Can you work these out from the drawing? Everything is in mm from the part's minimum corner. Give positions to 0.01 mm unless a question says otherwise; leave off trailing zeros. Write each question's results on one line, items separated by ' | '. Start each with the question number.
Item 1: Suppose I cut it at A-A on y = 1.25. Count the separate pieces of the cut face and the enclosed holes in it, then the cut area to 3 significant figures.
Item 2: Will these pins go through, and if not, where does the flat tip stop? P1, Ø2.5, axis at x = 15, z = 32.5, coming from the -Y side; P2, Ø5, axis at x = 109.015, z = 79, coming from the -Y side.
Item 3: Please list where these lines run through material, in increasing order: line 1 along Z through (x, y) = (100, 1.1); line 2 along X through (y, z) = (1.15, 32); line 3 along Z through (x, y) = (99, 0.85).
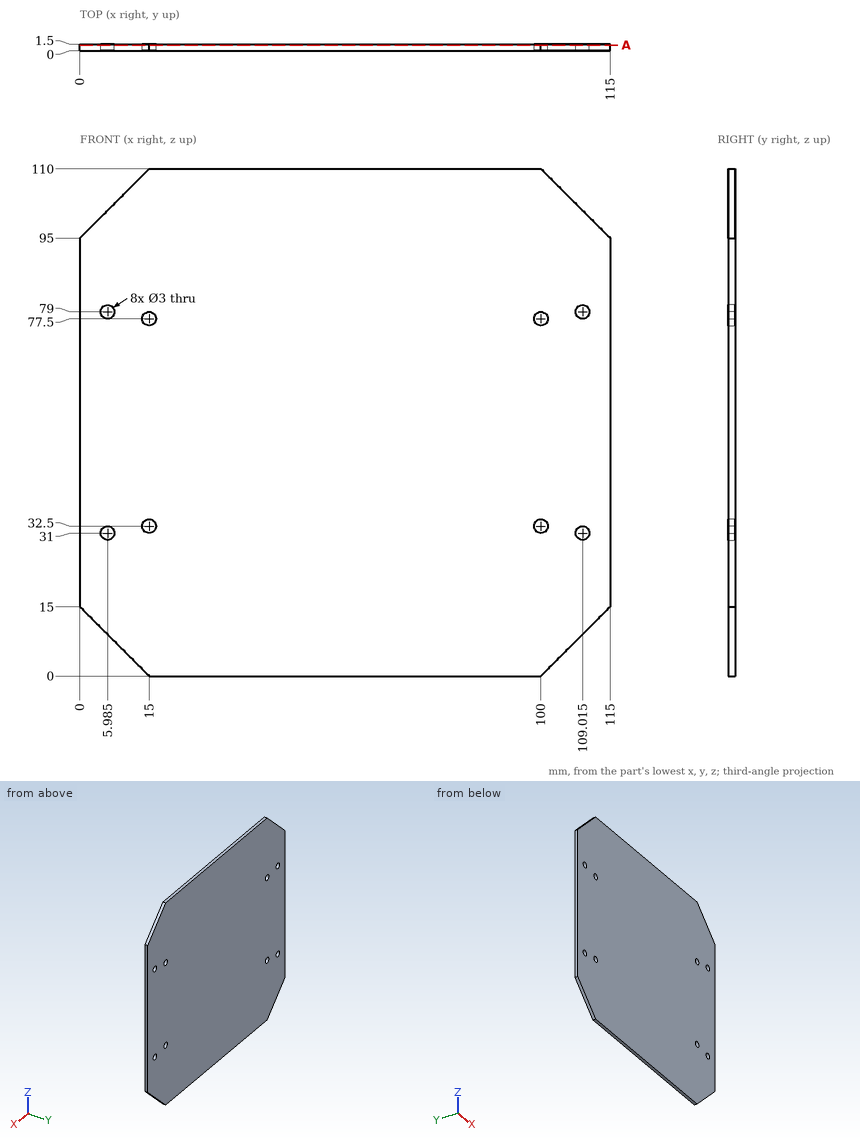
Checked values:
1) separate pieces: 1 | enclosed holes: 8 | area: 12,100 mm^2
2) P1: passes through | P2: stops at y = 0
3) line 1: z = 0 to 31, 34 to 76, 79 to 110 | line 2: x = 0 to 4.87, 7.1 to 13.59, 16.41 to 98.59, 101.41 to 107.9, 110.13 to 115 | line 3: z = 0 to 31.38, 33.62 to 76.38, 78.62 to 110
